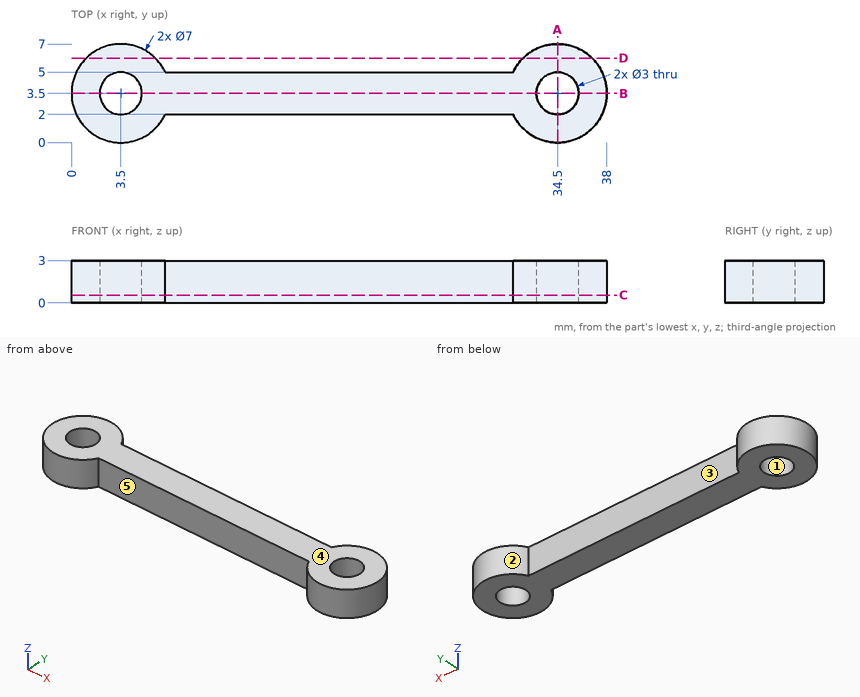
For this review, use the dimensioned drawing (mm, ordinates from the lowest corner) and the shaded views. A direction names the side the tool comes from. Round coordinates to 2 decimals unless told otherwise and drop trailing zeros. Order: outer loops, then holes, each group sorted by start corner. A loop starts at its lowest first (then second) coordinate and runs counter-clockwise, first axis right, second up. Notation, with made-up numbers: (63.25, 44.25) -> (93.25, 44.25) arc R26 cw to (93.25, 80.25) -> close; hole circle Ø9 at (60, 50.25). An arc over 180 degrees is marked (long way). Write item = value, one per line. Start each with the question number.
Item 1: Consider section A-A on x = 34.5. Write out the cut boundary in (y, z), plus the area to 3 significant figures.
Item 2: Consider section D-D on y = 6. Write out the cut boundary in (x, z), plus the area to 3 significant figures.
Item 3: Consider section B-B on y = 3.5. Write out the cut boundary in (x, z).
Item 4: For line 1 along Y through (x, z) = (3.5, 2.1); line 2 along X through (y, z) = (2.75, 1.75); line 3 along Y through (x, z) = (25, 0.4), list the stretches that pass through material, from the lowest coordinate up.
Item 5: For the marked faces 4 and 5, list the 3-axis set-ups (+Z, -Z, +X, -X, +Y, -Y) from which the entire face can be reached by the end or side of a thin tool; tool diameter is ignored.
Item 6: Mouldability with a two-part tool opening along Y and no side actions: class the marked faces 1, 2 and 3 as released by +Y, released by -Y, zero draft, split by the parting line, or undercut.
Item 7: Consider section C-C on z = 0.55. Write out the cut boundary in (x, y), plus the area to 3 significant figures.
Item 8: Clearance check with a flat-ended pin moving along its axis: pin 1 Ø1.5 at (x, z) = (19, 2.5) entering from +Y. State where the tip first meets the part, or that it passes through.
Conclusion:
q1.outline = (0, 0) -> (2, 0) -> (2, 3) -> (0, 3) -> close; (5, 0) -> (7, 0) -> (7, 3) -> (5, 3) -> close
q1.area = 12.0 mm2
q2.outline = (1.05, 0) -> (5.95, 0) -> (5.95, 3) -> (1.05, 3) -> close; (32.05, 0) -> (36.95, 0) -> (36.95, 3) -> (32.05, 3) -> close
q2.area = 29.4 mm2
q3.outline = (0, 0) -> (2, 0) -> (2, 3) -> (0, 3) -> close; (5, 0) -> (33, 0) -> (33, 3) -> (5, 3) -> close; (36, 0) -> (38, 0) -> (38, 3) -> (36, 3) -> close
q4.line_1 = 0 to 2, 5 to 7
q4.line_2 = 0.08 to 2.2, 4.8 to 33.2, 35.8 to 37.92
q4.line_3 = 2 to 5
q5.face_4 = +Z, +X, -X, +Y, -Y
q5.face_5 = +Z, -Z, -Y
q6.face_1 = undercut
q6.face_2 = split by the parting line
q6.face_3 = released by +Y
q7.outline = (6.66, 2) -> (31.34, 2) arc R3.5 ccw (long way) to (31.34, 5) -> (6.66, 5) arc R3.5 ccw (long way) to start; hole circle Ø3 at (3.5, 3.5); hole circle Ø3 at (34.5, 3.5)
q7.area = 135 mm2
q8.pin_1 = 5
